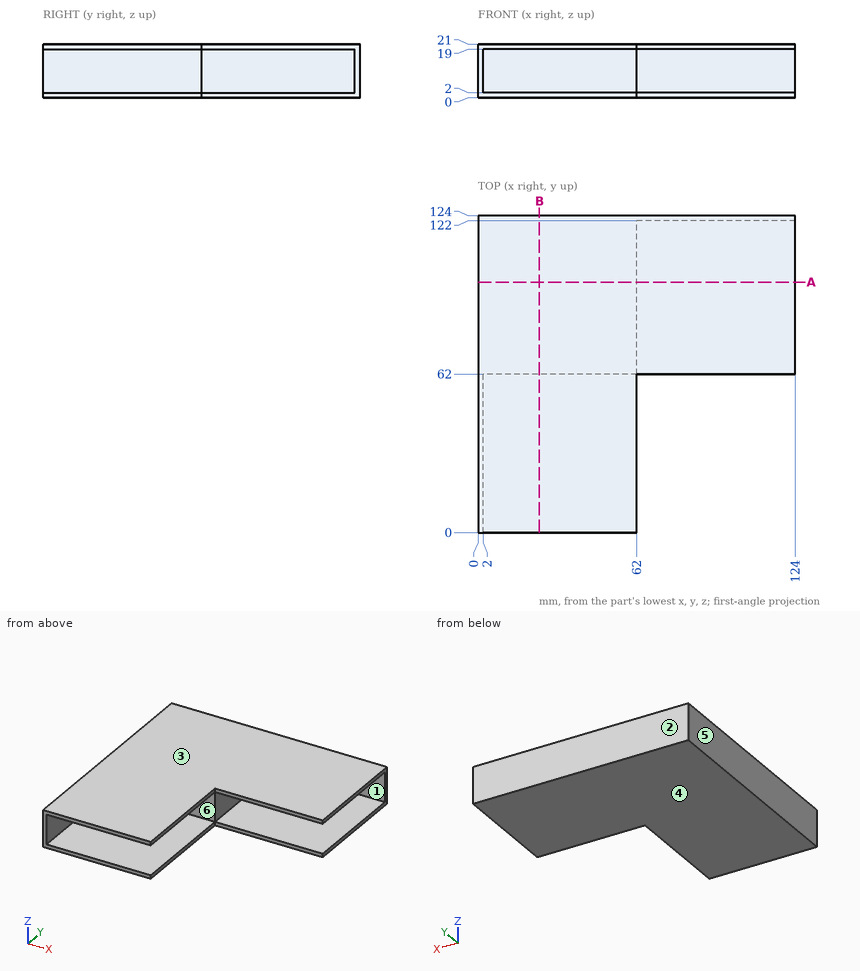
Can you work these out from the drawing? Everything is in mm from the part's minimum corner. A direction names the side the tool comes from. Give positions to 0.01 mm unless a question says otherwise; leave off trailing zeros. Order: outer loops, then holes, each group sorted by start corner. A loop starts at its lowest first (then second) coordinate and runs counter-clockwise, first axis right, second up. Notation, with made-up numbers: M 47,-17.5 L 55,-17.5 A32 cw 55,11.5 Z; hole C 42,-34 d10. An arc over 180 degrees is marked long. Write item = value, one per line. Start each with the question number.
Q1. Suppose I cut it at B-B (x = 24). Write out the boundary of the cut face in (y, z), plus the area to 3 significant figures.
Q2. We'd pull the mould along Z, two halves only. Please class the marked faces 1, 2, 3 and 4: pulls with the +Z half, pulls with the -Z half, needs draft (parallel to the pull), parting line crosses it, or undercut.
Q3. I need wall thicknesses on probe 1 along Z at (x, y) = (86, 81.5); probe 2 along Y at (x, z) = (116.5, 14.5); probe 3 along Y at (x, z) = (37, 18.25). Which ranges of each line are inside material? Lowest first, please. Write a range as [from, to].
Q4. Suppose I cut it at A-A (y = 98). Write out the boundary of the cut face in (x, z), plus the area to 3 significant figures.
Q5. Will these pins go through, and if not, where does the flat tip stop? pin 1 Ø1.6 at (x, z) = (83.5, 20) entering from -Y; pin 2 Ø3 at (y, z) = (78, 13.5) entering from -X; pin 3 Ø5 at (x, z) = (105.5, 11) entering from -Y; pin 4 Ø1 at (y, z) = (33.5, 1) entering from +X.
Q6. For the marked faces 5 and 6, which set-ups out of +Z, -Z, +X, -X, +Y, -Y let a thin tool reach every point of the face, with its end or its side?
Check result:
q1.outline = M 0,0 L 124,0 L 124,21 L 0,21 L 0,19 L 62,19 L 62,2 L 0,2 Z
q1.area = 1,550 mm2
q2.face_1 = undercut
q2.face_2 = needs draft
q2.face_3 = pulls with the +Z half
q2.face_4 = pulls with the -Z half
q3.probe_1 = [0, 2], [19, 21]
q3.probe_2 = [122, 124]
q3.probe_3 = [62, 124]
q4.outline = M 0,0 L 124,0 L 124,2 L 62,2 L 62,19 L 124,19 L 124,21 L 0,21 Z
q4.area = 1,550 mm2
q5.pin_1 = 62
q5.pin_2 = 0
q5.pin_3 = 122
q5.pin_4 = 62
q6.face_5 = +Z, -Z, -X, +Y, -Y
q6.face_6 = +X, -Y
